Build history of the part. All positions in model axes, mm. Round coordinates to 2 decimals unless told otherwise and drop trailing zeros. Order: outer loops, then holes, each group sorted by start corner. A loop starts at its lowest first (then second) coordinate and runs counter-clockwise, first axis right, second up. Notation, with made-up numbers: (82, -18) -> (124, -18) arc R32 cw to (124, 12) -> close; hole circle Ø4 at (73.5, 62). An arc over 180 degrees is marked (long way). Answer as a JSON object with one key per item and string values.
Autodesk Fusion 360 part; units mm, degrees
sketch "Skizze1" plane through (0, 0, 0) normal (0, 0, 1) x (1, 0, 0)
  line L0 (-2.1362, 3.7) -> (-4.2724, 0)
  line L1 (-4.2724, 0) -> (-2.1362, -3.7)
  line L2 (-2.1362, -3.7) -> (2.1362, -3.7)
  line L3 (2.1362, -3.7) -> (4.2724, 0)
  line L4 (4.2724, 0) -> (2.1362, 3.7)
  line L5 (2.1362, 3.7) -> (-2.1362, 3.7)
  dimension "d1" = 7.4
extrude "Extrusion1" add sketch "Skizze1" along normal blind 2
fillet "Abrundung1" radius 0.25 1 faces at (-0.7121, -1.2333, 2)
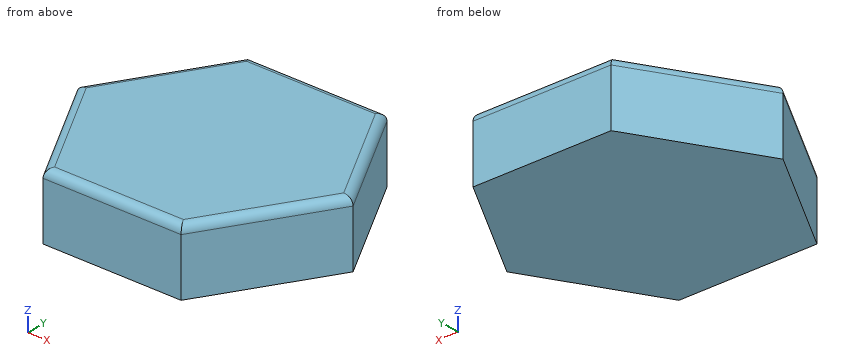
1) Cut at A-A, the plane z = 1.2. Give the cut face in (x, y), plus the area to 3 significant figures.
Checked values:
{"outline": "(-4.27, 0) -> (-2.14, -3.7) -> (2.14, -3.7) -> (4.27, 0) -> (2.14, 3.7) -> (-2.14, 3.7) -> close", "area": "47.4 mm²"}
2) Probe L1, parallel to X at y = -0.25, z = 1.15; L2, parallel to X at y = 3, z = 0.25; L3, parallel to Y at x = 4, z = 1.6. List the from-to ranges inside material, lowest first. Write a range as from..to.
Checked values:
{"L1": "x = -4.13..4.13", "L2": "x = -2.54..2.54", "L3": "y = -0.47..0.47"}
3) Flat gauge pin, fed straight in: pin 1 Ø1 at (y, z) = (-3, 0.5) entering from -X. Where does the tip first touch, or does it go through?
Checked values:
{"pin 1": "stops at x = -2.83"}
